Autodesk Inventor part; units mm, degrees
ref_plane "YZ Plane" through (0, 0, 0) normal (1, 0, 0) x (0, 1, 0)
ref_plane "XZ Plane" through (0, 0, 0) normal (0, 1, 0) x (-1, 0, 0)
ref_plane "XY Plane" through (0, 0, 0) normal (0, 0, 1) x (1, 0, 0)
sketch "Skizze1" plane through (0, 0, 0) normal (0, 0, 1) x (1, 0, 0)
  line L0 (-16, 20) -> (16, 20)
  line L1 (16, 20) -> (16, -20)
  line L2 (16, -20) -> (-16, -20)
  line L3 (-16, -20) -> (-16, 20)
  line L4 (-16, 20) -> (16, -20) construction
  line L5 (16, 20) -> (-16, -20) construction
  point P0 (0, 0)
  dimension "d0" = 32
  dimension "d1" = 40
extrude "Extrusion1" add sketch "Skizze1" along normal blind 15
sketch "Skizze2" plane through (-16, -20, 0) normal (0, -1, 0) x (1, 0, 0)
  line L0 (0, 15) -> (32, 15)
  line L1 (0, 0) -> (0, 15)
  line L2 (32, 0) -> (0, 0)
  line L3 (32, 0) -> (32, 15)
  line L4 (32, 15) -> (0, 15)
  circle A0 centre (16, 15) radius 10
  point P0 (16, 0)
  dimension "d4" = 20
extrude "Extrusion2" cut sketch "Skizze2" against normal blind 15 contours A0 L0 | L0 A0
sketch "Skizze3" plane through (-16, -5, 0) normal (0, -1, 0) x (1, 0, 0)
  line L0 (0, 0) -> (0, 15)
  line L1 (32, 0) -> (0, 0)
  line L2 (32, 0) -> (32, 15)
  line L3 (26, 15) -> (32, 15)
  line L4 (0, 15) -> (6, 15)
  line L5 (6, 15) -> (26, 15)
  circle A0 centre (16, 15) radius 10.5
  point P0 (16, 0)
  dimension "d7" = 21
extrude "Extrusion3" cut sketch "Skizze3" against normal blind 5 contours A0 L3 L5 L4 | L4 L5 L3 A0
sketch "Skizze4" plane through (-16, 0, 0) normal (0, -1, 0) x (1, 0, 0)
  line L0 (5.5, 15) -> (26.5, 15)
  circle A0 centre (16, 15) radius 12.5
  point P0 (16, 0)
  dimension "d10" = 25
extrude "Extrusion4" cut sketch "Skizze4" against normal through all
sketch "Skizze5" plane through (0, 0, 15) normal (0, 0, 1) x (1, 0, 0)
  line L0 (-16, 20) -> (-16, -20)
  line L1 (-16, -20) -> (-10, -20)
  line L2 (-10, -20) -> (-10, -5)
  line L3 (10, -5) -> (10, -20)
  line L4 (10, -20) -> (16, -20)
  line L5 (16, -20) -> (16, 20)
  circle A0 centre (-13, -13) radius 1.8
  circle A1 centre (13, -13) radius 1.8
  point P0 (0, 0)
  dimension "d13" = 3.6
  dimension "d14" = 3.6
  dimension "d15" = 7
  dimension "d16" = 7
  dimension "d17" = 3
  dimension "d18" = 3
extrude "Extrusion5" cut sketch "Skizze5" against normal through all
sketch "Skizze6" plane through (0, 0, 0) normal (0, 0, -1) x (-1, 0, 0)
  line L0 (-7.5, 7.5) -> (7.5, 7.5)
  line L1 (7.5, 7.5) -> (7.5, -7.5)
  line L2 (7.5, -7.5) -> (-7.5, -7.5)
  line L3 (-7.5, -7.5) -> (-7.5, 7.5)
  line L4 (-7.5, 7.5) -> (7.5, -7.5) construction
  line L5 (7.5, 7.5) -> (-7.5, -7.5) construction
  point P0 (0, 0)
  dimension "d21" = 15
  dimension "d22" = 15
extrude "Extrusion6" add sketch "Skizze6" along normal blind 20
sketch "Skizze7" plane through (0, 0, -20) normal (0, 0, -1) x (-1, 0, 0)
  circle A0 centre (0, 0) radius 2.3
  dimension "d25" = 4.6
extrude "Extrusion7" cut sketch "Skizze7" against normal blind 7
sketch "Skizze8" plane through (0, 0, 0) normal (0, 0, -1) x (-1, 0, 0)
  line L0 (12.5, 20) -> (16, 20)
  line L1 (16, 20) -> (16, 11.5)
  line L2 (16, 20) -> (16, -20)
  line L3 (16, 11.5) -> (-16, 11.5)
  line L4 (-16, 20) -> (-16, -20)
  line L5 (16, 20) -> (-16, 20)
  line L6 (-16, 20) -> (16, 20)
  point P0 (0, 0)
  dimension "d28" = 8.5
extrude "Extrusion8" cut sketch "Skizze8" along normal mid plane 58.75
properties part number "unterteil"
Work out the finished part from the listing and answer in its coordinate system (mm). A direction names the side the tool comes from. Give positions to 0.01 mm unless a question says otherwise; leave off trailing zeros. Order: outer loops, then holes, each group sorted by start corner. A loop starts at its lowest first (then second) coordinate and runs counter-clockwise, first axis right, second up. Notation, with made-up numbers: M 24,51 L 81,51 A27 cw 81,85 Z; hole C -13,-28.75 d7. An arc over 180 degrees is marked long. Return JSON: item names as keys, results as strings.
Q1. Find the intervals of material crossed by line 1 along Y through (x, z) = (13, 6); line 2 along Y through (x, z) = (0, -17.5); line 3 along Y through (x, z) = (4.5, -7.5), in increasing order. Write a range as [from, to].
Answer below:
{"line 1": "y = [-20, -14.8], [-11.2, 11.5]", "line 2": "y = [-7.5, -2.3], [2.3, 7.5]", "line 3": "y = [-7.5, 7.5]"}
Q2. Find section D-D, the plane x = 0. Write down the section's boundary in (y, z), and give its area (3 significant figures).
Answer below:
{"outline": "M -20,0 L -7.5,0 L -7.5,-20 L -2.3,-20 L -2.3,-13 L 2.3,-13 L 2.3,-20 L 7.5,-20 L 7.5,0 L 11.5,0 L 11.5,2.5 L 0,2.5 L 0,4.5 L -5,4.5 L -5,5 L -20,5 Z", "area": "394 mm^2"}
Q3. Find section C-C, the plane y = 9.5. Write down the section's boundary in (x, z).
Answer below:
{"outline": "M -16,0 L 16,0 L 16,15 L 12.5,15 A12.5 cw -12.5,15 L -16,15 Z"}
Q4. Find section B-B, the plane z = -14. Write down the section's boundary in (x, y).
Answer below:
{"outline": "M -7.5,-7.5 L 7.5,-7.5 L 7.5,7.5 L -7.5,7.5 Z; hole C 0,0 d4.6"}
Q5. Which of the six approach directions +Z, -Z, +X, -X, +Y, -Y give full straight-line access (tool end or side, diameter ignored) to faces 4 (the face through (7.5, 0, -10)), 5 (the face through (-7.5, 0, -10)), 6 (the face through (-0.2, -2.5, 4.5)), 7 (the face through (1.825, -1.4, -16.549)), 8 (the face through (0, 7.5, -10))?
Answer below:
{"face 4": "-Z, +X, +Y, -Y", "face 5": "-Z, -X, +Y, -Y", "face 6": "+Z, +Y", "face 7": "-Z", "face 8": "-Z, +X, -X, +Y"}
Q6. The mould has two halves that part along X. Classify faces 1 (the face through (0, -13, 5)), 2 (the face through (14, -4, 15)), 3 (the face through (-16, -4, 7)): pulls with the +X half, pulls with the -X half, needs draft (parallel to the pull), parting line crosses it, or undercut.
Answer below:
{"face 1": "undercut", "face 2": "needs draft", "face 3": "pulls with the -X half"}
Q7. Find section A-A, the plane x = -13. Write down the section's boundary in (y, z).
Answer below:
{"outline": "M -20,0 L -14.8,0 L -14.8,15 L -20,15 Z; M -11.2,0 L 11.5,0 L 11.5,15 L -11.2,15 Z"}
Q8. Each of these flat-tipped pins is pushed along its axis until it touches: pin 1 (4 mm diameter, centred on x = 4, z = 8, fed in from +Y); pin 2 (1 mm diameter, centred on x = 7, y = 4, fed in from +Z); pin 3 (3 mm diameter, centred on x = -13, y = -13, fed in from -Z); pin 4 (12 mm diameter, centred on y = 2, z = -13.5, fed in from +X). Where does it stop, or does it pass through?
Answer below:
{"pin 1": "stops at y = -5", "pin 2": "stops at z = 5", "pin 3": "passes through", "pin 4": "stops at x = 7.5"}
